Autodesk Inventor part; units mm, degrees
ref_plane "YZ Plane" through (0, 0, 0) normal (1, 0, 0) x (0, 1, 0)
ref_plane "XZ Plane" through (0, 0, 0) normal (0, 1, 0) x (-1, 0, 0)
ref_plane "XY Plane" through (0, 0, 0) normal (0, 0, 1) x (1, 0, 0)
sketch "Boceto1" plane through (0, 0, 0) normal (0, 0, 1) x (1, 0, 0)
  line L0 (0, 0) -> (9, 0) construction
  line L1 (9, 0) -> (9, 33)
  line L2 (42, 0) -> (42, 27)
  line L3 (42, 27) -> (33, 27)
  line L4 (33, 27) -> (33, 33)
  line L5 (33, 33) -> (9, 33)
  line L6 (42, 0) -> (42, 3) construction
  line L7 (42, 3) -> (40, 3) construction
  line L8 (40, 3) -> (37, 0)
  line L9 (40, 3) -> (43.5355, 3) construction
  line L10 (40, 3) -> (40, 0)
  line L11 (9, 0) -> (37, 0)
  line L12 (40, 0) -> (42, 0)
  line L13 (0, 0) -> (0, 41.2707) construction
  dimension "d0" = 9
  dimension "d1" = 33
  dimension "d2" = 33
  dimension "d3" = 27
  dimension "d4" = 9
  dimension "d5" = 3
  dimension "d6" = 2
  dimension "d7" = 135
  dimension "d8" = 6
revolve "Revolución1" add sketch "Boceto1" angle 360 about axis through (0, 0, 0) along (0, 1, 0)
properties part number "6_Piston"
Read the model definition and answer for the solid it produces. Units are mm, in the model's axes. A direction names the side the tool comes from. Coordinates: 2 decimals unless noted, no trailing zeros. Loops run counter-clockwise (first coordinate to the right, second up) from the corner with the lowest first, then second, coordinate; pieces in that order, holes last.
Q1. Each of these flat-tipped pins is pushed along its axis until it touches: pin 1 Ø1 at (y, z) = (6, -28.5) entering from +X; pin 2 Ø1 at (y, z) = (23, 30.5) entering from -X; pin 3 Ø1 at (y, z) = (10.5, 31) entering from -X. Where does it stop, or does it pass through?
Q2. Consider probe 1 along X at (y, z) = (13, 0); probe 2 along Z at (x, y) = (-0.5, 15); probe 3 along Z at (x, y) = (-12.5, 2.5). Determine where each line is inside the solid, lowest interval first.
Q3. The part is cut by section D-D on y = 26. Write down the section's boundary in (x, z).
Q4. The part is cut by section C-C on y = 2. Write down the section's boundary in (x, z).
Q5. The part is cut by section A-A on z = 0. Write down the section's boundary in (x, y).
Q6. The part is cut by section B-B on x = 0. Write down the section's boundary in (y, z).
Q7. Which of the six approach directions +Z, -Z, +X, -X, +Y, -Y give full straight-line access (tool end or side, diameter ignored) to faces 5 (the face through (30.5, 30, 12.6)), 6 (the face through (-1.172, 16.731, -8.923))?
Q8. The mould has two halves that part along X. Classify faces 1 (the face through (-25, 27, 22)), 2 (the face through (40.06, 13.69, -12.62)), 3 (the face through (-8.67, 1.48, -39.05)), 4 (the face through (19.99, 0.19, -31.36)): +X half, -X half, draft (parallel to the pull), parting line (faces both ways), or undercut.
Results below:
1. pin 1: stops at x = 31.3
1. pin 2: stops at x = -29.39
1. pin 3: stops at x = -28.87
2. probe 1: x = -42 to -9, 9 to 42
2. probe 2: z = -42 to -8.99, 8.99 to 42
2. probe 3: z = -40.1 to -38, -37.47 to 37.47, 38 to 40.1
3. outline: circle Ø84 at (0, 0); hole circle Ø18 at (0, 0)
4. outline: circle Ø84 at (0, 0); circle Ø78 at (0, 0); hole circle Ø80 at (0, 0); hole circle Ø18 at (0, 0)
5. outline: (-42, 0) - (-40, 0) - (-40, 3) - (-37, 0) - (-9, 0) - (-9, 33) - (-33, 33) - (-33, 27) - (-42, 27) - close; (9, 0) - (37, 0) - (40, 3) - (40, 0) - (42, 0) - (42, 27) - (33, 27) - (33, 33) - (9, 33) - close
6. outline: (0, -42) - (27, -42) - (27, -33) - (33, -33) - (33, -9) - (0, -9) - (0, -37) - (3, -40) - (0, -40) - close; (0, 9) - (33, 9) - (33, 33) - (27, 33) - (27, 42) - (0, 42) - (0, 40) - (3, 40) - (0, 37) - close
7. face 5: +Y
7. face 6: +Y, -Y
8. face 1: draft
8. face 2: parting line
8. face 3: undercut
8. face 4: undercut
